The drawing under review shows one solid part. Ordinate dimensions are in mm from its lowest x, y, z. Give positions to 0.01 mm unless a question says otherwise; leave off trailing zeros. Write each loop counter-clockwise with the first axis right and the second up, starting at its lowest first coordinate (ties: lowest second). Pieces come first, ordered by that corner, then holes. Notation, with made-up numbers: (9.25, 73.5) -> (57.25, 73.5) arc R29 cw to (57.25, 95.5) -> close; hole circle Ø10 at (-12, 52). An arc over 180 degrees is marked (long way). Write item = value, one per line.
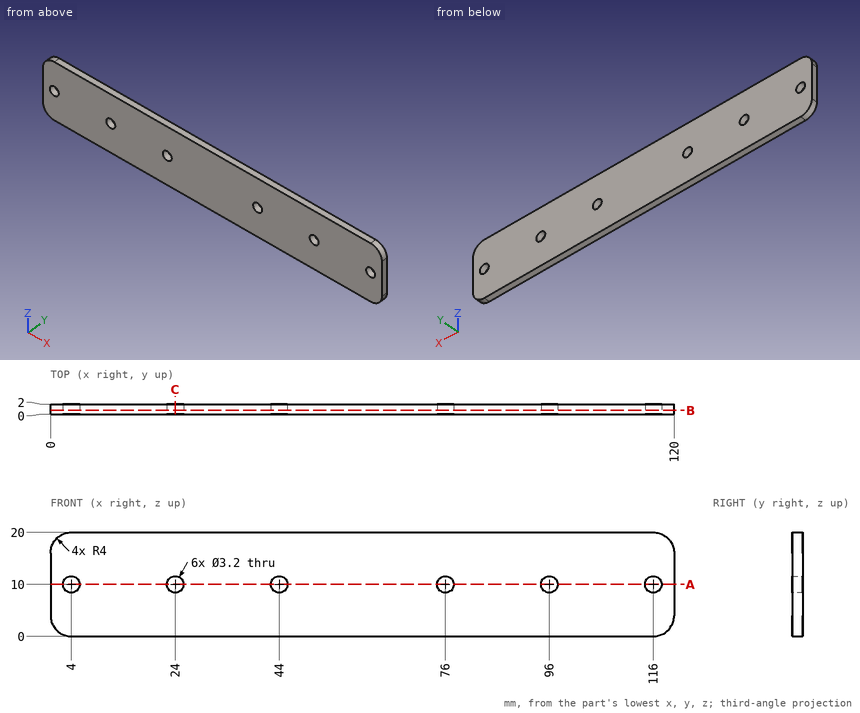
(1) Take a section at C-C (x = 24). Write out the cut boundary in (y, z).
Answers below:
outline = (0, 0) -> (2, 0) -> (2, 8.4) -> (0, 8.4) -> close; (0, 11.6) -> (2, 11.6) -> (2, 20) -> (0, 20) -> close
(2) Take a section at A-A (z = 10). Write out the cut boundary in (x, y).
Answers below:
outline = (0, 0) -> (2.4, 0) -> (2.4, 2) -> (0, 2) -> close; (5.6, 0) -> (22.4, 0) -> (22.4, 2) -> (5.6, 2) -> close; (25.6, 0) -> (42.4, 0) -> (42.4, 2) -> (25.6, 2) -> close; (45.6, 0) -> (74.4, 0) -> (74.4, 2) -> (45.6, 2) -> close; (77.6, 0) -> (94.4, 0) -> (94.4, 2) -> (77.6, 2) -> close; (97.6, 0) -> (114.4, 0) -> (114.4, 2) -> (97.6, 2) -> close; (117.6, 0) -> (120, 0) -> (120, 2) -> (117.6, 2) -> close
(3) Take a section at B-B (y = 0.75). Write out the cut boundary in (x, z).
Answers below:
outline = (0, 4) arc R4 ccw to (4, 0) -> (116, 0) arc R4 ccw to (120, 4) -> (120, 16) arc R4 ccw to (116, 20) -> (4, 20) arc R4 ccw to (0, 16) -> close; hole circle Ø3.2 at (4, 10); hole circle Ø3.2 at (24, 10); hole circle Ø3.2 at (44, 10); hole circle Ø3.2 at (76, 10); hole circle Ø3.2 at (96, 10); hole circle Ø3.2 at (116, 10)
(4) To check wall thickness, follow probe 1 along Z at (x, y) = (96, 1.4); probe 2 along X at (y, z) = (0.95, 18.25); probe 3 along X at (y, z) = (1.8, 3). State the ranges of each line that lie inside material, in increasing order.
Answers below:
probe_1 = 0 to 8.4, 11.6 to 20
probe_2 = 0.69 to 119.31
probe_3 = 0.13 to 119.87
